The listing builds one solid part. Answer for the finished solid, in the listing's coordinates (mm). Face numbers are marked on the shaded views. A direction names the side the tool comes from. Give positions to 0.01 mm unless a question says otherwise; leave off trailing zeros. Write each loop counter-clockwise with the first axis right and the second up, starting at its lowest first coordinate (ties: lowest second). Pieces come first, ordered by that corner, then holes. Notation, with made-up numbers: M 83,9 L 88,9 A16 ccw 88,29 Z; hole C 47,74 d4. An arc over 180 degrees is marked long. Answer as a JSON object with one key per item and string values.
Autodesk Inventor part; units mm, degrees
ref_plane "YZ Plane" through (0, 0, 0) normal (1, 0, 0) x (0, 1, 0)
ref_plane "XZ Plane" through (0, 0, 0) normal (0, 1, 0) x (-1, 0, 0)
ref_plane "XY Plane" through (0, 0, 0) normal (0, 0, 1) x (1, 0, 0)
sketch "スケッチ1" plane through (0, 0, 0) normal (0, 0, 1) x (1, 0, 0)
  circle A0 centre (0, 0) radius 40
  line L0 (0, 0) -> (0, 40)
  line L1 (-40, 0) -> (0, 0)
  dimension "d0" = 80
extrude "押し出し1" add sketch "スケッチ1" along normal mid plane 5 contours L0 L1 A0 picked at (-23.4047, 12.51)
sketch "スケッチ2" plane through (0, 0, 2.5) normal (0, 0, 1) x (1, 0, 0)
  line L0 (0, 0) -> (0, 40)
  arc A0 (0, 40) -> (-40, 0) centre (0, 0) ccw
  line L1 (-40, 0) -> (0, 0)
  line L2 (-40, 0) -> (0, 0)
  line L3 (0, 0) -> (0, -5)
  line L4 (0, -5) -> (-40, -5)
  line L5 (-40, -5) -> (-40, 0)
  line L6 (0, -5) -> (5, -5)
  line L7 (5, -5) -> (5, 5)
  line L8 (5, 5) -> (0, 5)
  line L9 (0, 5) -> (0, -5)
  dimension "d3" = 5
  dimension "d4" = 5
  dimension "d5" = 10
extrude "押し出し2" add sketch "スケッチ2" against normal blind 5 contours L3 L4 L5 L1 | L0 L8 L7 L6 L3
sketch "スケッチ3" plane through (0, 0, 2.5) normal (0, 0, 1) x (1, 0, 0)
  circle A0 centre (0, 0) radius 35
  point P0 (-35, 0)
  point P1 (-34.0566, 8.0716)
  point P2 (-31.2771, 15.708)
  point P3 (-26.8116, 22.4976)
  dimension "d8" = 70
  dimension "d11" = 40
hole "穴1" at (0, 0, 2.5) at (-35, 0, 2.5) at (-34.0566, 8.0716, 2.5) at (-31.2771, 15.708, 2.5) at (-26.8116, 22.4976, 2.5) direction (0, 0, -1) diameter 3.4 end through all
sketch "スケッチ4" plane through (0, 0, 2.5) normal (0, 0, 1) x (1, 0, 0)
  arc A0 (-1.7, 0) -> (-1.7, 0) centre (0, 0) ccw
  circle A1 centre (0, 0) radius 30
  circle A2 centre (-26.8116, 22.4976) radius 1.7
  circle A3 centre (-31.2771, 15.708) radius 1.7
  circle A4 centre (-34.0566, 8.0716) radius 1.7
  circle A5 centre (-35, 0) radius 1.7
  circle A6 centre (0, 0) radius 1.7
  line L0 (0, 5) -> (0, 40)
  arc A7 (0, 40) -> (-40, 0) centre (0, 0) ccw
  line L1 (-40, 0) -> (-40, -5)
  line L2 (-40, -5) -> (5, -5)
  line L3 (5, -5) -> (5, 5)
  line L4 (5, 5) -> (0, 5)
  line L5 (0, 0) -> (-30.6418, 25.7115)
  line L6 (-30.6418, 25.7115) -> (-22.9813, 19.2836)
  line L7 (-22.9813, 19.2836) -> (-19.7674, 23.1139)
  line L8 (-19.7674, 23.1139) -> (-27.4278, 29.5417)
  line L9 (-27.4278, 29.5417) -> (-30.6418, 25.7115)
  line L10 (0, 5) -> (-29.5804, 5)
  point P0 (-27.1875, 29.3401)
  dimension "d20" = 60
  dimension "d21" = 40
  dimension "d22" = 5
extrude "押し出し3" cut sketch "スケッチ4" against normal blind 55 contours L10 A1 L5 | L5 A1 L0 L10 | L7 L8 A7 L0 A1
sketch "スケッチ7" plane through (0, 0, 2.5) normal (0, 0, 1) x (1, 0, 0)
  line L0 (-40, -5) -> (5, -5)
  line L1 (-40, -5) -> (-30, -5)
  line L2 (-30, -5) -> (-30, -25)
  line L3 (-30, -25) -> (-40, -25)
  line L4 (-40, -25) -> (-40, -5)
  line L5 (-30, -25) -> (5, -5)
  point P0 (0, 0)
  dimension "d40" = 10
  dimension "d41" = 20
extrude "押し出し5" add sketch "スケッチ7" against normal blind 5
sketch "スケッチ8" plane through (0, 0, 2.5) normal (0, 0, 1) x (1, 0, 0)
  line L0 (-40, 0) -> (-40, -25)
  line L1 (-40, -25) -> (-30, -25)
  point P0 (0, 0)
  point P1 (-35, -10)
  point P2 (-35, -20)
  dimension "d44" = 5
  dimension "d45" = 5
  dimension "d46" = 10
  dimension "d47" = 5
hole "穴3" at (-35, -20, 2.5) at (-35, -10, 2.5) direction (0, 0, -1) diameter 3.4 end through all
sketch "スケッチ9" plane through (0, 0, 2.5) normal (0, 0, 1) x (1, 0, 0)
  circle A0 centre (0, 0) radius 1.7
  circle A1 centre (0, 0) radius 5
  line L0 (-29.5804, 5) -> (5, 5)
  circle A2 centre (-35, -20) radius 1.7
  circle A3 centre (-35, -20) radius 5
  line L1 (-40, -25) -> (-40, 0)
  line L2 (-35, -20) -> (0, 0) construction
  line L3 (-32.5193, -24.3412) -> (2.4807, -4.3412)
  line L4 (-2.4807, 4.3412) -> (-37.4807, -15.6588)
  arc A4 (-37.4807, -15.6588) -> (-32.5193, -24.3412) centre (-35, -20) ccw
  arc A5 (2.4807, -4.3412) -> (-2.4807, 4.3412) centre (0, 0) ccw
  circle A6 centre (-35, -10) radius 1.7
  circle A7 centre (-35, -20) radius 1.7
  line L5 (-19.7674, 23.1139) -> (-27.1875, 29.3401)
  arc A8 (-27.1875, 29.3401) -> (-40, 0) centre (0, 0) ccw
  line L6 (-40, 0) -> (-40, -25)
  line L7 (-40, -25) -> (-30, -25)
  line L8 (-30, -25) -> (5, -5)
  line L9 (5, -5) -> (5, 5)
  line L10 (5, 5) -> (-29.5804, 5)
  arc A9 (-22.9813, 19.2836) -> (-29.5804, 5) centre (0, 0) ccw
  line L11 (-22.9813, 19.2836) -> (-19.7674, 23.1139)
  circle A10 centre (-26.8116, 22.4976) radius 1.7
  circle A11 centre (-31.2771, 15.708) radius 1.7
  circle A12 centre (-34.0566, 8.0716) radius 1.7
  circle A13 centre (-35, 0) radius 1.7
  circle A14 centre (0, 0) radius 1.7
  circle A15 centre (-26.8116, 22.4976) radius 5
  point P0 (-17.5, -10)
  point P1 (5, 0)
  point P2 (2.4807, -4.3412)
  point P3 (-35, -25)
  point P4 (0, 5)
  point P5 (-40, -20)
  point P6 (-22.9813, 19.2836)
  point P7 (-23.5976, 26.3278)
  point P8 (-30.6418, 25.7115)
extrude "押し出し6" cut sketch "スケッチ9" against normal blind 5 contours A1 L9 L8 L7 A3 L3 | L0 L9 A1 | A3 L7 L1 | A15 L5 L11 | A8 L5 A15
fillet "フィレット1" radius 2 1 edges at (-29.5804, 5, 0)
properties part number "side_part"
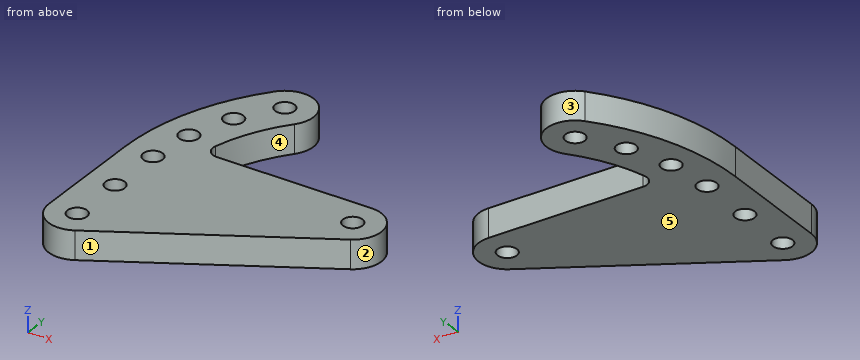
1. For the marked faces 4 and 5, determine the directions among +Z, -Z, +X, -X, +Y, -Y from which every point of the face is accessible in a straight line to the end or side of a thin tool.
Verdict:
{"face 4": "+Z, -Z, +X", "face 5": "-Z, +X, -X, +Y, -Y"}
2. Flat-ended cylindrical pins translate along their axes: pin 1 (1 mm diameter, centred on x = -33.5, z = -0.5, fed in from +Y); pin 2 (3 mm diameter, centred on y = -19, z = 0.5, fed in from +X); pin 3 (3 mm diameter, centred on x = -32.5, z = -1, fed in from -Y). Find the tip coordinate at first contact, or state that the pin passes through.
Verdict:
{"pin 1": "stops at y = 22.61", "pin 2": "stops at x = -20.55", "pin 3": "stops at y = -24.9"}
3. A cutting plane is placed at B-B, the plane y = 23.5. Give the vertices of the cut face in (x, z).
Verdict:
{"outline": "M -32.37,-2.5 L -28.18,-2.5 L -28.18,2.5 L -32.37,2.5 Z; M -25.44,-2.5 L -21.91,-2.5 L -21.91,2.5 L -25.44,2.5 Z"}
4. Consider line 1 along X through (y, z) = (0, 0); line 2 along X through (y, z) = (0.5, 0); line 3 along Y through (x, z) = (-35, 1.4). Determine where each line is inside the solid, lowest interval first.
Verdict:
{"line 1": "x = -40 to -36.7, -33.3 to -1.7, 1.7 to 5", "line 2": "x = -40 to -36.62, -33.38 to -1.62, 1.62 to 4.97", "line 3": "y = -25 to -21.7, -18.3 to -11.7, -8.3 to -1.7, 1.7 to 6.66, 9.49 to 19.36"}
5. A cutting plane is placed at A-A, the plane x = -35. Give the vertices of the cut face in (y, z), plus the area to 3 significant figures.
Verdict:
{"outline": "M -25,-2.5 L -21.7,-2.5 L -21.7,2.5 L -25,2.5 Z; M -18.3,-2.5 L -11.7,-2.5 L -11.7,2.5 L -18.3,2.5 Z; M -8.3,-2.5 L -1.7,-2.5 L -1.7,2.5 L -8.3,2.5 Z; M 1.7,-2.5 L 6.66,-2.5 L 6.66,2.5 L 1.7,2.5 Z; M 9.49,-2.5 L 19.36,-2.5 L 19.36,2.5 L 9.49,2.5 Z", "area": "157 mm2"}
6. A cutting plane is placed at D-D, the plane y = 3. Give the vertices of the cut face in (x, z).
Verdict:
{"outline": "M -39.89,-2.5 L 4,-2.5 L 4,2.5 L -39.89,2.5 Z"}
7. A cutting plane is placed at C-C, the plane z = 0.45. Give the vertices of the cut face in (x, y), plus the area to 3 significant figures.
Verdict:
{"outline": "M -40,-20 A5 ccw -32.52,-24.34 L 2.48,-4.34 A5 ccw 0,5 L -27.11,5 A2 cw -29.05,7.5 A30 cw -22.98,19.28 A5 ccw -30.64,25.71 A40 ccw -40,0 Z; hole C -35,-20 d3.4; hole C -35,-10 d3.4; hole C -35,0 d3.4; hole C -34.06,8.07 d3.4; hole C -31.28,15.71 d3.4; hole C -26.81,22.5 d3.4; hole C 0,0 d3.4", "area": "1,080 mm2"}
8. The mould has two halves that part along Y. Classify the marked faces 1, 2 and 3: released by +Y, released by -Y, zero draft, split by the parting line, or undercut.
Verdict:
{"face 1": "released by -Y", "face 2": "split by the parting line", "face 3": "undercut"}
